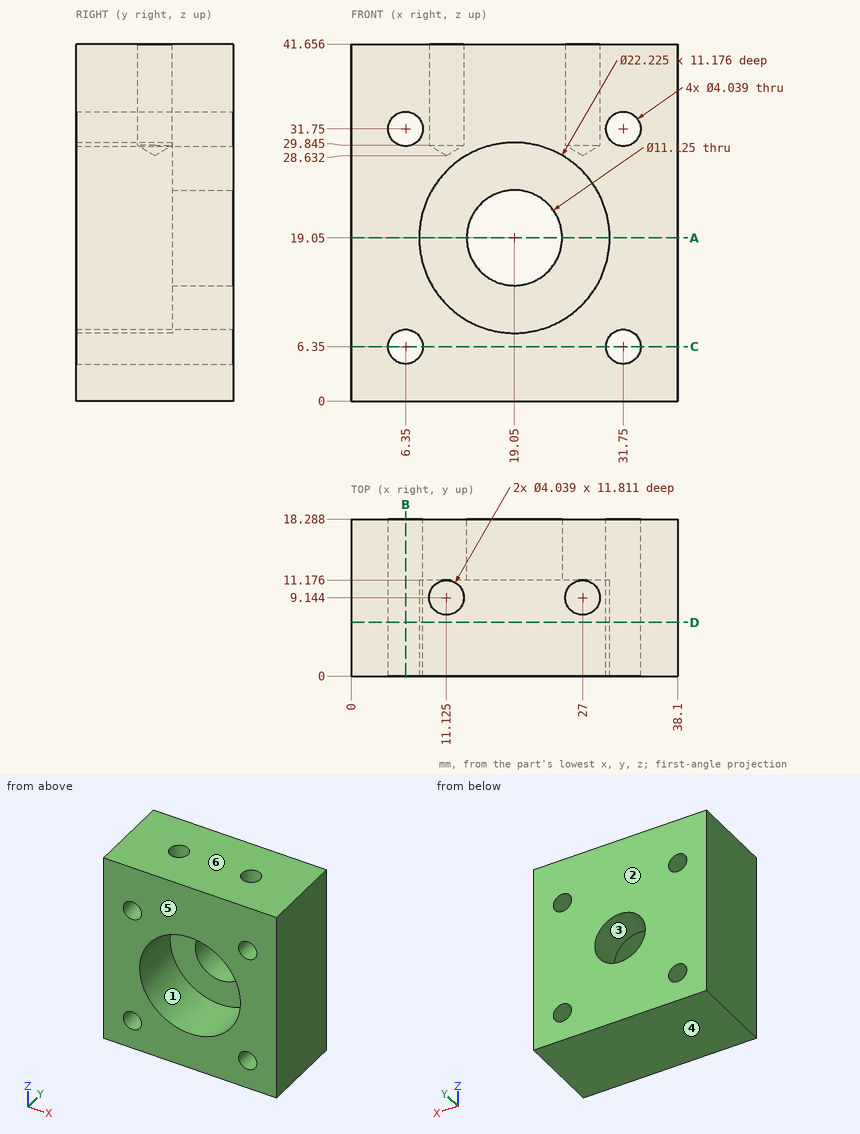
Print and shaded views of the part. All mm, measured from the part's lowest x, y and z. A direction names the side the tool comes from. Coordinates: 2 decimals unless noted, no trailing zeros. Order: outer loops, then holes, each group sorted by start corner. A loop starts at its lowest first (then second) coordinate and runs counter-clockwise, first axis right, second up. Notation, with made-up numbers: M 47,39 L 55,39 A19 ccw 55,51 Z; hole C -39.75,-36.75 d7. An arc over 180 degrees is marked long. Answer as CSV lines item,"result".
1) Drill centre lines: L1, parallel to Z at x = 19.05, y = 5; L2, parallel to Z at x = 6, y = 14.5 (1 decimal); L3, parallel to Z at x = 19.05, y = 13.75. Where is each one in solid material? Low to high. Write a range as from..to.
Verdict:
L1,"0..7.94, 30.16..41.66"
L2,"0..4.4, 8.3..29.8, 33.7..41.7"
L3,"0..13.49, 24.61..41.66"
2) Cut at B-B (x = 6.35). List the corners of the cut face in (y, z).
Verdict:
outline,"M 0,0 L 18.29,0 L 18.29,4.33 L 0,4.33 Z; M 0,8.37 L 18.29,8.37 L 18.29,29.73 L 0,29.73 Z; M 0,33.77 L 18.29,33.77 L 18.29,41.66 L 0,41.66 Z"
3) Mould opens along Z. For the marked faces 3, 4, 5 and 6 say: released by +Z, released by -Z, zero draft, split by the parting line, or undercut.
Verdict:
face 3,"undercut"
face 4,"released by -Z"
face 5,"zero draft"
face 6,"released by +Z"
4) 3-axis set-ups, long thin cutter, end or side, ignore diameter. For the marked faces 1 and 2: which of +Z, -Z, +X, -X, +Y, -Y reach the whole face in a straight line?
Verdict:
face 1,"-Y"
face 2,"+Z, -Z, +X, -X, +Y"
5) Cut at D-D (y = 6.25). Give the number of separate pieces and of enclosed holes in the cut face, then the cut area to 3 significant figures.
Verdict:
separate pieces,"1"
enclosed holes,"5"
area,"1,150 mm2"
6) Cut at C-C (z = 6.35). List the corners of the cut face in (x, y).
Verdict:
outline,"M 0,0 L 4.33,0 L 4.33,18.29 L 0,18.29 Z; M 8.37,0 L 29.73,0 L 29.73,18.29 L 8.37,18.29 Z; M 33.77,0 L 38.1,0 L 38.1,18.29 L 33.77,18.29 Z"
7) Flat gauge pins, fed straight in: P1, Ø3, axis at x = 27, y = 9.14, coming from the +Z side (1 decimal); P2, Ø6.5, axis at x = 19.05, z = 19.05, coming from the +Y side; P3, Ø18, axis at x = 19.05, z = 19.05, coming from the -Y side. Where does each tip first touch, or does it go through?
Verdict:
P1,"z = 29.5"
P2,"through"
P3,"y = 11.18"
8) Cut at A-A (z = 19.05). List the corners of the cut face in (x, y).
Verdict:
outline,"M 0,0 L 7.94,0 L 7.94,11.18 L 13.49,11.18 L 13.49,18.29 L 0,18.29 Z; M 24.61,11.18 L 30.16,11.18 L 30.16,0 L 38.1,0 L 38.1,18.29 L 24.61,18.29 Z"
